The model under review builds one solid part; all positions refer to its coordinate system, in mm. A direction names the side the tool comes from. Give positions to 0.01 mm unless a question says otherwise; leave off trailing zeros. Write each loop counter-clockwise with the first axis right and the second up, starting at its lowest first coordinate (ties: lowest second). Pieces come first, ordered by that corner, then holes. Notation, with made-up numbers: (12.25, 9) - (53.25, 9) arc R10 ccw to (53.25, 13) - close; hole circle Ø9 at (40.25, -20). An arc over 180 degrees is marked (long way). Write item = value, one per line.
```python
from build123d import *

# Parameters (mm, degrees)
SKETCH_1_R          = 12
EXTRUDE_1_DEPTH     = 3.9
SKETCH_2_R          = 13
EXTRUDE_2_DEPTH     = 1.1
SKETCH_3_R          = 7.5
CUT_EXTRUDE_1_DEPTH = 5


with BuildPart() as part:
    # 草图1 → 凸台-拉伸1 (new body)
    with BuildSketch(Plane(origin=(0, 0, 0), x_dir=(1, 0, 0), z_dir=(0, 1, 0))):
        Circle(SKETCH_1_R)
    extrude(amount=EXTRUDE_1_DEPTH)

    # 草图2 → 凸台-拉伸2 (add)
    with BuildSketch(Plane(origin=(0, 3.9, 0), x_dir=(1, 0, 0), z_dir=(0, 1, 0))):
        Circle(SKETCH_2_R)
    extrude(amount=EXTRUDE_2_DEPTH)

    # 草图3 → 切除-拉伸1 (cut)
    with BuildSketch(Plane.XZ):
        Circle(SKETCH_3_R)
    extrude(amount=-CUT_EXTRUDE_1_DEPTH, mode=Mode.SUBTRACT)


solid = part.part
```
1. Machinability: for faces 1 (the flat face through (9, 3.9, 9)), 2 (the flat face through (5, 0, -6)), which of the approach directions +Z, -Z, +X, -X, +Y, -Y give a long, thin tool a straight path to every point of the face, cutting with its end or side? Answer none if there is none.
Findings below:
face_1 = -Y
face_2 = +Z, -Z, +X, -X, -Y
2. For line 1 (Z direction, x = 0, y = 3.55); line 2 (Z direction, x = 1.5, y = 4.15); line 3 (X direction, y = 1.05, z = 2), list the stretches that pass through material, from the lowest coordinate up. Write a range as from..to.
Findings below:
line_1 = -12..-7.5, 7.5..12
line_2 = -12.91..-7.35, 7.35..12.91
line_3 = -11.83..-7.23, 7.23..11.83
3. Take a section at B-B on z = 0. Give the boundary of the cut face in (x, y), and give its area (3 significant figures).
Findings below:
outline = (-13, 3.9) - (-12, 3.9) - (-12, 0) - (-7.5, 0) - (-7.5, 5) - (-13, 5) - close; (7.5, 0) - (12, 0) - (12, 3.9) - (13, 3.9) - (13, 5) - (7.5, 5) - close
area = 47.2 mm²
4. Take a section at C-C on y = 1.25. Give the boundary of the cut face in (x, z), and give its area (3 significant figures).
Findings below:
outline = circle Ø24 at (0, 0); hole circle Ø15 at (0, 0)
area = 276 mm²
5. Draft analysis for pull direction X (two halves, no side actions). For faces 3 (the cylindrical face through (-7.493, 2.465, 0.33)), 4 (the cylindrical face through (-10.316, 4.442, 7.91)), 5 (the flat face through (6, 5, 6)), state which applies: +X half, -X half, draft (parallel to the pull), parting line (faces both ways), or undercut.
Findings below:
face_3 = undercut
face_4 = parting line
face_5 = draft
6. Insertion check: P1, Ø2, axis at y = 3, z = -1.5, coming from the -X side; P2, Ø2, axis at x = -2.5, y = 3.5, coming from the +Z side; P3, Ø3, axis at y = 1.5, z = -7, coming from the -X side. Each pin has a flat end and moves straight along its axis. Give the tip position at first contact, or say it passes through.
Findings below:
P1 = -12.96
P2 = 12.9
P3 = -10.67
7. Take a section at A-A on x = 0. Give the boundary of the cut face in (y, z).
Findings below:
outline = (0, -12) - (3.9, -12) - (3.9, -13) - (5, -13) - (5, -7.5) - (0, -7.5) - close; (0, 7.5) - (5, 7.5) - (5, 13) - (3.9, 13) - (3.9, 12) - (0, 12) - close
8. Take a section at D-D on x = -10. Give the boundary of the cut face in (y, z), and give its area (3 significant figures).
Findings below:
outline = (0, -6.63) - (3.9, -6.63) - (3.9, -8.31) - (5, -8.31) - (5, 8.31) - (3.9, 8.31) - (3.9, 6.63) - (0, 6.63) - close
area = 70.0 mm²
